Geometry check sheet. Reference: the model listing, model coordinates, mm. A direction names the side the tool comes from. Give positions to 0.01 mm unless a question says otherwise; leave off trailing zeros. Write each loop counter-clockwise with the first axis right and the second up, starting at its lowest first coordinate (ties: lowest second). Pieces come first, ordered by that corner, then holes. Notation, with made-up numbers: (3, 31.25) - (27, 31.25) arc R29 cw to (27, 62.25) - close; hole circle Ø1 at (-16.75, -39). An arc over 180 degrees is marked (long way). Use a Markdown table: item, result.
```python
from build123d import *

# Parameters (mm, degrees)
SKETCH_1_W          = 77
SKETCH_1_H          = 58.5
EXTRUDE_1_DEPTH     = 2
SKETCH_2_W          = 77
SKETCH_2_H          = 58.5
SKETCH_2_W_2        = 73
SKETCH_2_H_2        = 54
EXTRUDE_2_DEPTH     = 11
CUT_EXTRUDE_1_REACH = 85.388
SKETCH_3_W          = 9
SKETCH_3_H          = 11
SKETCH_3_W_2        = 11


with BuildPart() as part:
    # 草图1 → 凸台-拉伸1 (new body)
    with BuildSketch(Plane(origin=(0, 0, 0), x_dir=(1, 0, 0), z_dir=(0, 1, 0))):
        Rectangle(SKETCH_1_W, SKETCH_1_H)
    extrude(amount=EXTRUDE_1_DEPTH)

    # 草图2 → 凸台-拉伸2 (add)
    with BuildSketch(Plane(origin=(0, 2, 0), x_dir=(1, 0, 0), z_dir=(0, 1, 0))):
        Rectangle(SKETCH_2_W, SKETCH_2_H)
        with Locations((0, 0.25)):
            Rectangle(SKETCH_2_W_2, SKETCH_2_H_2, mode=Mode.SUBTRACT)
    extrude(amount=EXTRUDE_2_DEPTH)

    # 草图3 → 切除-拉伸1 (cut, up to next)
    with BuildSketch(Plane.ZY.offset(38.5), mode=Mode.PRIVATE) as cut_extrude_1_sk1:
        with Locations((18.25, 7.5)):
            Rectangle(SKETCH_3_W, SKETCH_3_H)
    cut_extrude_1_tool1 = extrude(cut_extrude_1_sk1.sketch, amount=-CUT_EXTRUDE_1_REACH, mode=Mode.PRIVATE) & part.part
    # 草图3 → 切除-拉伸1 (cut, up to next)
    with BuildSketch(Plane.ZY.offset(38.5), mode=Mode.PRIVATE) as cut_extrude_1_sk2:
        with Locations((-21.75, 7.5)):
            Rectangle(SKETCH_3_W_2, SKETCH_3_H)
    cut_extrude_1_tool2 = extrude(cut_extrude_1_sk2.sketch, amount=-CUT_EXTRUDE_1_REACH, mode=Mode.PRIVATE) & part.part
    add(cut_extrude_1_tool1.solids().sort_by_distance((-38.5, 7.5, 18.25))[0], mode=Mode.SUBTRACT)
    add(cut_extrude_1_tool2.solids().sort_by_distance((-38.5, 7.5, -21.75))[0], mode=Mode.SUBTRACT)


solid = part.part
```
1) Section check D-D on z = 16. Record the boundary of the cut face in (x, y), then the cut area to 3 significant figures.
Working result:
| item | result |
|---|---|
| outline | (-38.5, 0) - (38.5, 0) - (38.5, 13) - (36.5, 13) - (36.5, 2) - (-38.5, 2) - close |
| area | 176 mm² |
2) Mould release check, pull along X, two halves, no side actions. Record for faces 4 (the flat face through (38.5, 6, 0)), 5 (the flat face through (-38.5, 6, 7)), 6 (the flat face through (36.5, 7, 0)), 7 (the flat face through (-1, 6, 29.25)): pulls with the +X half, pulls with the -X half, needs draft (parallel to the pull), parting line crosses it, or undercut.
Working result:
| item | result |
|---|---|
| face 4 | pulls with the +X half |
| face 5 | pulls with the -X half |
| face 6 | undercut |
| face 7 | needs draft |
3) Depth check by flat-ended pin: P1, Ø16, axis at x = 4.5, z = -11, coming from the +Y side; P2, Ø10, axis at x = -7, z = -15, coming from the -Y side. Enter the tip coordinate at first touch or a pass-through.
Working result:
| item | result |
|---|---|
| P1 | stops at y = 2 |
| P2 | stops at y = 0 |
4) Set-up check for faces 1 (the flat face through (-38, 7, -16.25)), 2 (the flat face through (-38, 13, -1)), 3 (the flat face through (-1, 7, 26.75)): record each of +Z, -Z, +X, -X, +Y, -Y from which the full face is reachable in a straight line by a thin tool's end or side.
Working result:
| item | result |
|---|---|
| face 1 | -X, +Y |
| face 2 | +Z, -Z, +X, -X, +Y |
| face 3 | +Y |
5) Section check B-B on x = -14.5. Record the boundary of the cut face in (y, z).
Working result:
| item | result |
|---|---|
| outline | (0, -29.25) - (13, -29.25) - (13, -27.25) - (2, -27.25) - (2, 26.75) - (13, 26.75) - (13, 29.25) - (0, 29.25) - close |
6) Section check A-A on y = 3.25. Record the boundary of the cut face in (x, z).
Working result:
| item | result |
|---|---|
| outline | (-38.5, -29.25) - (38.5, -29.25) - (38.5, 29.25) - (-38.5, 29.25) - (-38.5, 22.75) - (-36.5, 22.75) - (-36.5, 26.75) - (36.5, 26.75) - (36.5, -27.25) - (-38.5, -27.25) - close; (-38.5, -16.25) - (-36.5, -16.25) - (-36.5, 13.75) - (-38.5, 13.75) - close |
7) Material ranges on L1, parallel to X at y = 10.5, z = 10; L2, parallel to Z at x = -31.5, y = 6.25; L3, parallel to Y at x = -5, z = 13, recorded low to high. Write a range as from..to.
Working result:
| item | result |
|---|---|
| L1 | x = -38.5..-36.5, 36.5..38.5 |
| L2 | z = -29.25..-27.25, 26.75..29.25 |
| L3 | y = 0..2 |
8) Section check C-C on z = -12. Record the boundary of the cut face in (x, y).
Working result:
| item | result |
|---|---|
| outline | (-38.5, 0) - (38.5, 0) - (38.5, 13) - (36.5, 13) - (36.5, 2) - (-36.5, 2) - (-36.5, 13) - (-38.5, 13) - close |
